```python
from build123d import *

# Parameters (mm, degrees)
EXTRUDE_THIN1_DEPTH = 46


with BuildPart() as part:
    # Sketch3 → Extrude-Thin1 (new body)
    with BuildSketch(Plane.ZY.offset(-268.297)):
        Polygon((3, -16.39), (28.524751964, -16.39), (28.524751964, -47.39), (3, -47.39), (3, -49.39), (30.524751964, -49.39), (30.524751964, -14.39), (3, -14.39), align=None)
    extrude(amount=EXTRUDE_THIN1_DEPTH)


solid = part.part
```
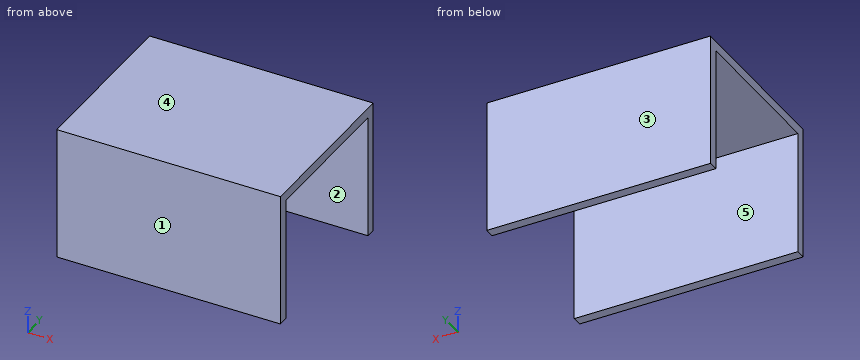
Source: CAD feature listing. Evaluate the final solid. Frame: model axes, mm. Face numbers are marked on the shaded views. A direction names the side the tool comes from. Coordinates: 2 decimals unless noted, no trailing zeros. Loops run counter-clockwise (first coordinate to the right, second up) from the corner with the lowest first, then second, coordinate; pieces in that order, holes last. Notation, with made-up numbers: M 84,-12.75 L 102,-12.75 A20 cw 102,-3.75 Z; hole C 8,48 d4. An arc over 180 degrees is marked long. Use a Markdown table: item, result. Add a question column.
Q1. Section query C-C, the plane y = -45. Return loops of the section in (x, z), and give its area (3 significant figures).
Q2. Material intervals for L1, parallel to Y at x = 237, z = 16; L2, parallel to Z at x = 231.5, y = -33, sorted ascending.
Q3. Section query A-A, the plane z = 19. Return loops of the section in (x, y).
Q4. Section query B-B, the plane x = 249.5. Return loops of the section in (y, z), and give its area (3 significant figures).
Q5. Access query for the marked faces 4 and 5. Directions: +Z, -Z, +X, -X, +Y, -Y. A direction counts if a zero-diameter tool reaches every point of the face in a straight line with its end or side. Return the directions, or none.
Q6. First-contact query: pin 1 (1.5 mm diameter, centred on x = 263, y = -23, fed in from -Z). Flat tip, straight axial feed; report the tip coordinate or a pass-through.
Q7. Draft query along Y for the marked faces 1, 2 and 3. Return one class per face: pulls with the +Y half, pulls with the -Y half, needs draft (parallel to the pull), parting line crosses it, or undercut.
Result:
| question | item | result |
|---|---|---|
| 1 | outline | M 222.3,28.52 L 268.3,28.52 L 268.3,30.52 L 222.3,30.52 Z |
| 1 | area | 92.0 mm2 |
| 2 | L1 | y = -49.39 to -47.39, -16.39 to -14.39 |
| 2 | L2 | z = 28.52 to 30.52 |
| 3 | outline | M 222.3,-49.39 L 268.3,-49.39 L 268.3,-47.39 L 222.3,-47.39 Z; M 222.3,-16.39 L 268.3,-16.39 L 268.3,-14.39 L 222.3,-14.39 Z |
| 4 | outline | M -49.39,3 L -47.39,3 L -47.39,28.52 L -16.39,28.52 L -16.39,3 L -14.39,3 L -14.39,30.52 L -49.39,30.52 Z |
| 4 | area | 172 mm2 |
| 5 | face 4 | +Z, +X, -X, +Y, -Y |
| 5 | face 5 | -Z, +X, -X |
| 6 | pin 1 | stops at z = 28.52 |
| 7 | face 1 | pulls with the -Y half |
| 7 | face 2 | undercut |
| 7 | face 3 | pulls with the +Y half |
